Verification items for the finished model (mm, model axes). Face numbers are marked on the shaded views. A direction names the side the tool comes from. Give positions to 0.01 mm unless a question says otherwise; leave off trailing zeros. Write each loop counter-clockwise with the first axis right and the second up, starting at its lowest first coordinate (ties: lowest second). Pieces come first, ordered by that corner, then holes. Notation, with made-up numbers: (28, -12) -> (66, -12) arc R19 cw to (66, 12) -> close; hole circle Ø6 at (66, 89.25). An arc over 180 degrees is marked (long way). Answer as CSV lines item,"result". Start each with the question number.
1) Material ranges on L1, parallel to Z at x = 7, y = 3.75; L2, parallel to Y at x = 6.75, z = -65; L3, parallel to Y at x = 8.75, z = -25.5, recorded low to high.
2) Gauge pin test, flat ends, axial feed: pin 1 Ø2 at (x, z) = (4, -2.5) entering from -Y; pin 2 Ø1 at (x, y) = (4, -8.5) entering from +Z; pin 3 Ø3 at (x, z) = (6, -74) entering from +Y. Record the tip position at first contact, or that the pin passes through.
3) Tool access check on the marked faces 1, 2 and 3. Record the directions out of +Z, -Z, +X, -X, +Y, -Y that give a thin tool (end or side, any length) a straight path to the whole face; none if there is none.
4) Mould release check, pull along Y, two halves, no side actions. Record for the marked faces 4, 5, 6 and 7: released by +Y, released by -Y, zero draft, split by the parting line, or undercut.
5) Sectioned sample at D-D on y = 4.25. Record the cut outline in (x, z).
6) Sectioned sample at C-C on z = -69. Record the cut outline in (x, y), and give its area (3 significant figures).
7) Sectioned sample at A-A on z = -5. Record the cut outline in (x, y).
```python
from build123d import *

# Parameters (mm, degrees)
F1_DEPTH = 10
F2_R     = 7
F3_R     = 2
F4_R     = 5
F5_R     = 1.49999
F6_SIZE  = 1.99999
F7_R     = 1


# Not quite as in the source:
# - a fillet or chamfer is up to 0.001 mm smaller than in the source, because OpenCascade refuses the exact size


with BuildPart() as f1:
    # F0 (on Right) → F1 (new body)
    with BuildSketch(Plane.YZ):
        Polygon((0, -35), (0, 0), (9, 0), (9, -3), (5, -30), (9, -36.9282032303), (10.7320508076, -35.9282032303), (7.8850353118, -30.9970277416), (12, -3.2210160959), (12, 5), (-5, 5), (-5, -77), (-15, -77), (-15, -70), (-18, -70), (-18, -80), (-2, -80), (-2, -35), align=None)
    extrude(amount=F1_DEPTH)

    # F2
    f2_edges = [f1.edges().sort_by_distance(p)[0] for p in [
        (5, -5, -77),
    ]]
    fillet(f2_edges, radius=F2_R)

    # F3
    f3_edges = [f1.edges().sort_by_distance(p)[0] for p in [
        (5, -15, -77),
    ]]
    fillet(f3_edges, radius=F3_R)

    # F4
    f4_edges = [f1.edges().sort_by_distance(p)[0] for p in [
        (5, -5, 5),
        (5, 12, 5),
        (5, -18, -80),
        (5, -2, -80),
    ]]
    fillet(f4_edges, radius=F4_R)

    # F5 (radius 1.5 in the source; OpenCascade refuses exactly that, so slightly less here)
    f5_edges = [f1.edges().sort_by_distance(p)[0] for p in [
        (5, 9, -36.928203),
        (5, -18, -70),
        (5, -15, -70),
    ]]
    fillet(f5_edges, radius=F5_R)

    # F6 (size 2 in the source; OpenCascade refuses exactly that, so slightly less here)
    f6_edges = [f1.edges().sort_by_distance(p)[0] for p in [
        (5, 0, -35),
    ]]
    chamfer(f6_edges, length=F6_SIZE)

    # F7
    f7_edges = [f1.edges().sort_by_distance(p)[0] for p in [
        (5, 0, 0),
        (5, 9, 0),
    ]]
    fillet(f7_edges, radius=F7_R)


solid = f1.part
```
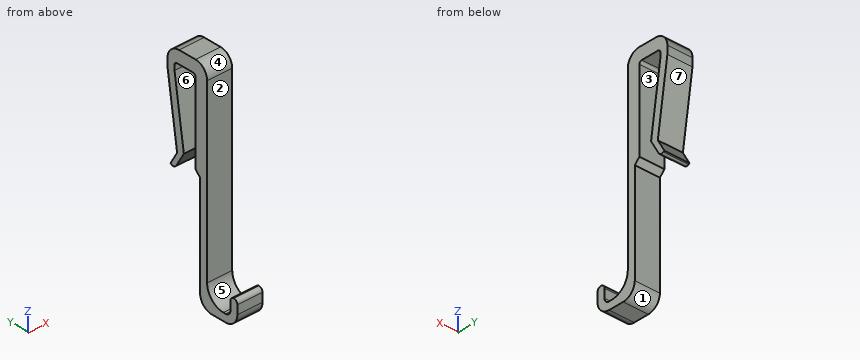
Ans:
1,L1,"z = 0 to 5"
1,L2,"y = -5 to -2"
1,L3,"y = -5 to 0, 5.67 to 8.7"
2,pin 1,"stops at y = -5"
2,pin 2,"stops at z = -75.74"
2,pin 3,"stops at y = -2"
3,face 1,"-Z, +X, -X, +Y"
3,face 2,"+Z, +X, -X, -Y"
3,face 3,"-Z, +X, -X"
4,face 4,"released by -Y"
4,face 5,"undercut"
4,face 6,"undercut"
4,face 7,"released by +Y"
5,outline,"(0, 0) -> (10, 0) -> (10, 5) -> (0, 5) -> close"
6,outline,"(0, -5) -> (10, -5) -> (10, -2) -> (0, -2) -> close"
6,area,"30.0 mm²"
7,outline,"(0, -5) -> (10, -5) -> (10, 0) -> (0, 0) -> close; (0, 8.7) -> (10, 8.7) -> (10, 11.74) -> (0, 11.74) -> close"
